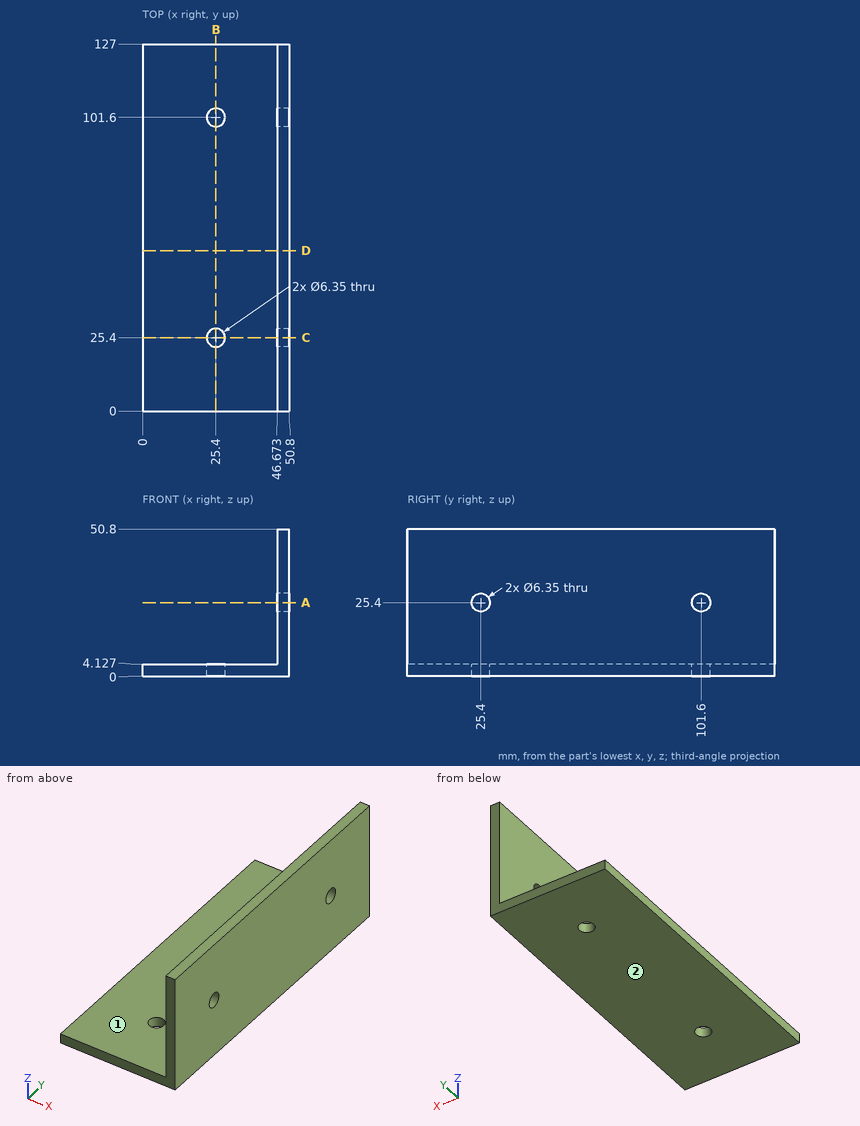
Drawing for the job (mm, zero at the part's lowest x, y, z). A direction names the side the tool comes from. Give positions to 0.01 mm unless a question says otherwise; leave off trailing zeros. Write each loop counter-clockwise with the first axis right and the second up, starting at its lowest first coordinate (ties: lowest second). Pieces come first, ordered by that corner, then holes. Notation, with made-up numbers: M 20.5,48 L 52.5,48 A20 cw 52.5,62 Z; hole C -23,-35.5 d5. An arc over 180 degrees is marked long. Return JSON: item names as keys, results as strings. Group by question number.
(1) Flat gauge pins, fed straight in: pin 1 Ø5 at (y, z) = (13, 20.5) entering from -X; pin 2 Ø23.5 at (x, y) = (21, 78) entering from +Z; pin 3 Ø5 at (x, y) = (25.4, 101.6) entering from -Z; pin 4 Ø10 at (x, y) = (25.4, 25.4) entering from -Z. Where does each tip first touch, or does it go through?
(2) 3-axis set-ups, long thin cutter, end or side, ignore diameter. For the marked faces 1 and 2: which of +Z, -Z, +X, -X, +Y, -Y reach the whole face in a straight line?
(3) Band-saw the part on A-A (z = 25.4). Give the cut face in (x, y) (1 decimal), and give its area (3 significant figures).
(4) Band-saw the part on C-C (y = 25.4). Give the cut face in (x, z) (1 decimal), and give its area (3 significant figures).
(5) Band-saw the part on D-D (y = 55.5). Give the cut face in (x, z).
(6) Drill centre lines: L1, parallel to Y at x = 25.4, z = 2.55 (1 decimal); L2, parallel to Z at x = 49.9, y = 25.4 (1 decimal); L3, parallel to X at y = 25, z = 2. Where is each one in solid material? Low to high. Write a range as [from, to].
(7) Band-saw the part on B-B (x = 25.4). Give the cut face in (y, z) (1 decimal), and give its area (3 significant figures).
Entries:
{
 "1": {"pin 1": "stops at x = 46.67", "pin 2": "stops at z = 4.13", "pin 3": "passes through", "pin 4": "stops at z = 0"},
 "2": {"face 1": "+Z, -X, +Y, -Y", "face 2": "-Z, +X, -X, +Y, -Y"},
 "3": {"outline": "M 46.7,0 L 50.8,0 L 50.8,22.2 L 46.7,22.2 Z; M 46.7,28.6 L 50.8,28.6 L 50.8,98.4 L 46.7,98.4 Z; M 46.7,104.8 L 50.8,104.8 L 50.8,127 L 46.7,127 Z", "area": "472 mm^2"},
 "4": {"outline": "M 0,0 L 22.2,0 L 22.2,4.1 L 0,4.1 Z; M 28.6,0 L 50.8,0 L 50.8,22.2 L 46.7,22.2 L 46.7,4.1 L 28.6,4.1 Z; M 46.7,28.6 L 50.8,28.6 L 50.8,50.8 L 46.7,50.8 Z", "area": "350 mm^2"},
 "5": {"outline": "M 0,0 L 50.8,0 L 50.8,50.8 L 46.67,50.8 L 46.67,4.13 L 0,4.13 Z"},
 "6": {"L1": "y = [0, 22.2], [28.6, 98.4], [104.8, 127]", "L2": "z = [0, 22.2], [28.6, 50.8]", "L3": "x = [0, 22.25], [28.55, 50.8]"},
 "7": {"outline": "M 0,0 L 22.2,0 L 22.2,4.1 L 0,4.1 Z; M 28.6,0 L 98.4,0 L 98.4,4.1 L 28.6,4.1 Z; M 104.8,0 L 127,0 L 127,4.1 L 104.8,4.1 Z", "area": "472 mm^2"}
}
